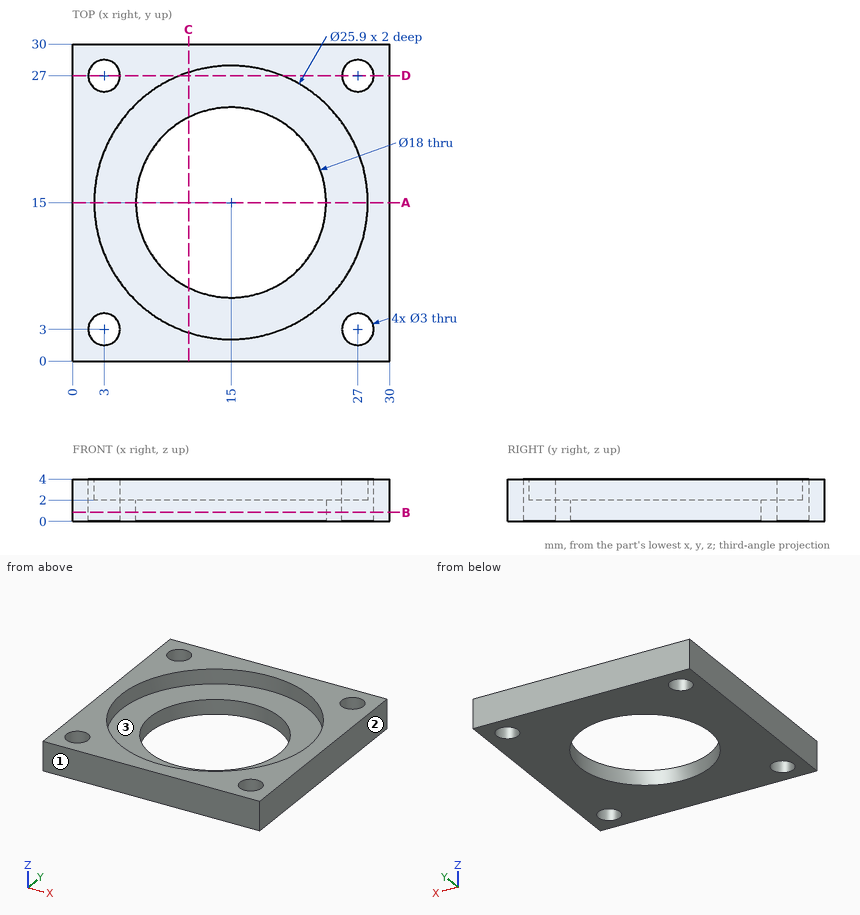
Study the drawing (mm; zero at the part's minimum x, y, z) and answer. Give positions to 0.01 mm unless a question says otherwise; leave off trailing zeros. Loops run counter-clockwise (first coordinate to the right, second up) from the corner with the lowest first, then second, coordinate; pieces in that order, holes last. Notation, with made-up numbers: (7.25, -24) -> (22.25, -24) arc R14 ccw to (22.25, 2) -> close; hole circle Ø10 at (85.25, 34). An arc over 180 degrees is marked (long way). Write item = value, one per line. Start each with the question number.
(1) Find section A-A on y = 15. Give the vertices of the cut face in (x, z), and give its area (3 significant figures).
(2) Find section D-D on y = 27. Give the vertices of the cut face in (x, z).
(3) Find the intervals of material crossed by probe 1 along Y at (x, z) = (3, 0.95); probe 2 along Y at (x, z) = (15, 0.55); probe 3 along Y at (x, z) = (15, 3.4), in increasing order. Write a range as from..to.
(4) The mould has two halves that part along X. Classify the marked faces 1, 2 and 3: +X half, -X half, draft (parallel to the pull), parting line (faces both ways), or undercut.
(5) Find section C-C on x = 11. Give the vertices of the cut face in (y, z).
(6) Given pin 1 Ø5 at (x, y) = (27, 3) entering from -Z, flat-ended and moving along its own axis, determine where the tip first touches the part or whether it passes through.
(7) Find section B-B on z = 0.85. Give the vertices of the cut face in (x, y).
From the geometry:
q1.outline = (0, 0) -> (6, 0) -> (6, 2) -> (2.05, 2) -> (2.05, 4) -> (0, 4) -> close; (24, 0) -> (30, 0) -> (30, 4) -> (27.95, 4) -> (27.95, 2) -> (24, 2) -> close
q1.area = 32.2 mm^2
q2.outline = (0, 0) -> (1.5, 0) -> (1.5, 4) -> (0, 4) -> close; (4.5, 0) -> (25.5, 0) -> (25.5, 4) -> (19.87, 4) -> (19.87, 2) -> (10.13, 2) -> (10.13, 4) -> (4.5, 4) -> close; (28.5, 0) -> (30, 0) -> (30, 4) -> (28.5, 4) -> close
q3.probe_1 = 0..1.5, 4.5..25.5, 28.5..30
q3.probe_2 = 0..6, 24..30
q3.probe_3 = 0..2.05, 27.95..30
q4.face_1 = draft
q4.face_2 = +X half
q4.face_3 = undercut
q5.outline = (0, 0) -> (6.94, 0) -> (6.94, 2) -> (2.68, 2) -> (2.68, 4) -> (0, 4) -> close; (23.06, 0) -> (30, 0) -> (30, 4) -> (27.32, 4) -> (27.32, 2) -> (23.06, 2) -> close
q6.pin_1 = 0
q7.outline = (0, 0) -> (30, 0) -> (30, 30) -> (0, 30) -> close; hole circle Ø3 at (3, 3); hole circle Ø3 at (3, 27); hole circle Ø18 at (15, 15); hole circle Ø3 at (27, 3); hole circle Ø3 at (27, 27)
